Design review of the part shown in the three views and the two pictorial views. Dimensions are in mm from the part's minimum x, y and z. A direction names the side the tool comes from. Round coordinates to 2 decimals unless told otherwise and drop trailing zeros. Loops run counter-clockwise (first coordinate to the right, second up) from the corner with the lowest first, then second, coordinate; pieces in that order, holes last.
1) Take a section at B-B (y = 21). State the section outline as (x, z) points (1 decimal), then the cut area to 3 significant figures.
2) Wall thickness on L1, parallel to Z at x = 14.75, y = 4.5 (1 decimal); L2, parallel to Z at x = 14.5, y = 10 (1 decimal); L3, parallel to Y at x = 9.75, z = 5.5 (1 decimal): over which ranges is each line inside the solid? List them lowest first.
3) Mouldability with a two-part tool opening along Z and no side actions: class the marked faces 4, 5, 6 and 7 as pulls with the +Z half, pulls with the -Z half, needs draft (parallel to the pull), parting line crosses it, or undercut.
4) Tool access review of the marked faces 1, 2 and 3: name each direction out of +Z, -Z, +X, -X, +Y, -Y from which nothing blocks a thin tool from reaching the whole face with its end or side.
5) Insertion check: pin 1 (8 mm diameter, centred on x = 7, z = 17.5, fed in from -Y); pin 2 (12 mm diameter, centred on y = 12.5, z = 15, fed in from -X); pin 3 (5 mm diameter, centred on x = 3, z = 3, fed in from +Y) (1 decimal); pin 4 (1 mm diameter, centred on y = 21, z = 14.5, fed in from +X) (1 decimal). Each pin has a flat end and moves straight along its axis. Give the tip position at first contact, or say it passes through.
6) Take a section at A-A (y = 13.5). State the section outline as (x, z) points (1 decimal).
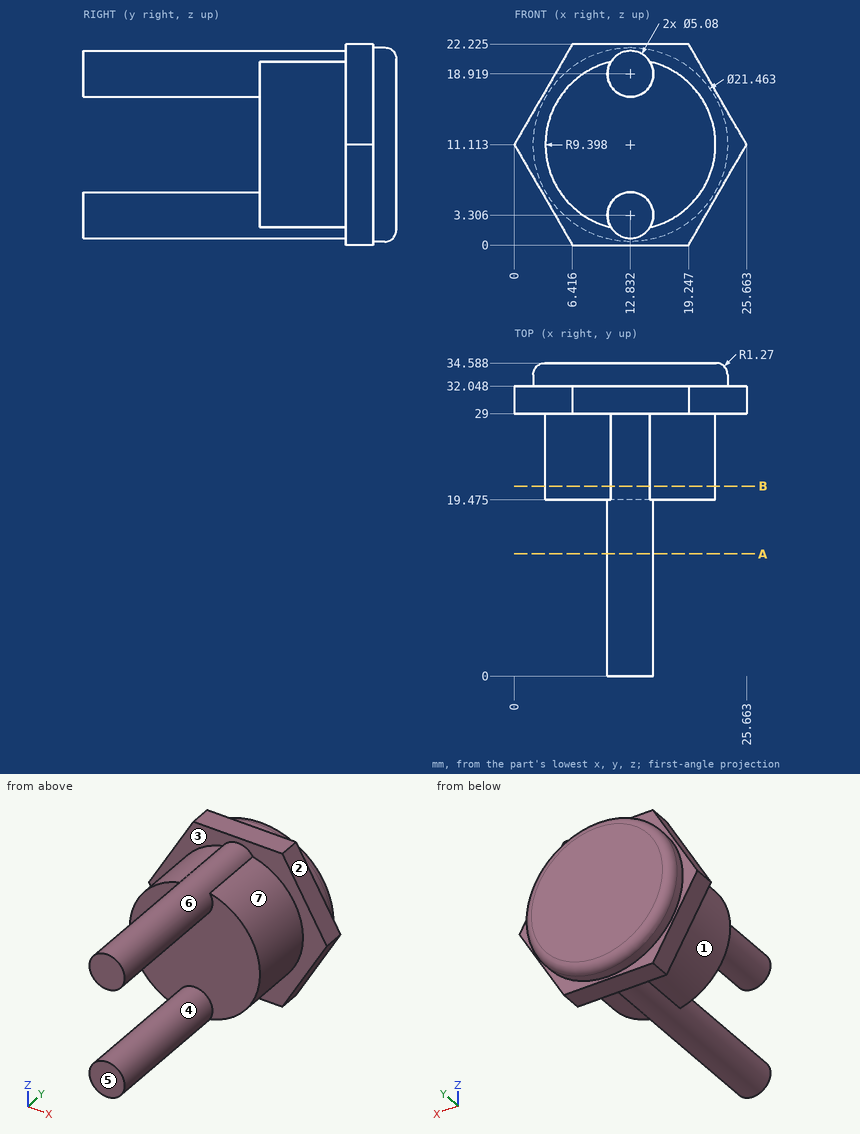
Response:
1. outline: (10.7, 2) arc R2.5 ccw to (15, 2) arc R9.4 ccw to (15, 20.3) arc R2.5 ccw to (10.7, 20.3) arc R9.4 ccw to start
1. area: 283 mm2
2. L1: z = 1.6 to 5, 17.3 to 20.6
2. L2: z = 1.4 to 5.2, 17 to 20.8
2. L3: y = 19.5 to 34.6
3. face 4: undercut
3. face 5: needs draft
3. face 6: undercut
3. face 7: parting line crosses it
4. face 1: -X, -Y
4. face 2: +Z, +X, +Y, -Y
4. face 3: -Y
5. pin 1: stops at y = 0
5. pin 2: stops at x = 10.29
5. pin 3: stops at y = 34.3
5. pin 4: stops at x = 21.8
6. outline: circle Ø5.1 at (12.8, 3.3); circle Ø5.1 at (12.8, 18.9)
